Here's how the part is built. I have some questions about the finished solid (model axes, mm). A direction names the side the tool comes from. Coordinates: 2 decimals unless noted, no trailing zeros. Write each loop counter-clockwise with the first axis right and the second up, starting at its lowest first coordinate (ties: lowest second). Pieces come first, ordered by that corner, then holes.
from build123d import *

# Parameters (mm, degrees)
F0_W      = 1.2
F0_H      = 9
F5_DEPTH  = 9
F7_DEPTH  = 1
F6_W      = 6
F6_H      = 1
F8_DEPTH  = 0.4
F9_DEPTH  = 1
F6_W_2    = 1
F6_H_2    = 1.2
F10_DEPTH = 1
F11_R     = 0.3
F13_DEPTH = 1
F14_DEPTH = 0.4
F15_SIZE  = 0.2


with BuildPart() as f2:
    # F2: sweep along a path in F1
    with BuildLine(Plane.XZ) as f2_path:
        Line((0, 0), (0, 1))
    # F0 (on Top) → F2 (sweep)
    with BuildSketch(Plane.XY):
        Polygon((-12, -8), (12, -8), (12, 1), (12, 8), (12, 9), (12, 17), (-12, 17), (-12, 9), (-12, 8), (-12, 1), align=None)
        with Locations((-12.6, -3.5)):
            Rectangle(F0_W, F0_H)
        with Locations((12.6, -3.5)):
            Rectangle(F0_W, F0_H)
    sweep(path=f2_path.line)

    # F3: sweep along a path in F1
    with BuildLine(Plane.XZ) as f3_path:
        Line((0, 0), (0, 1))
        Line((0, 1), (0, 4))
    # F0 (on Top) → F3 (sweep)
    with BuildSketch(Plane.XY):
        with Locations((-12.6, -3.5)):
            Rectangle(F0_W, F0_H)
        with Locations((12.6, -3.5)):
            Rectangle(F0_W, F0_H)
    sweep(path=f3_path.line)

    # F4 (on face) → F5 (join, through all)
    with BuildSketch(Plane.XZ.offset(8)):
        Polygon((-11.75, 1), (-12, 4), (-12, 1), align=None)
        Polygon((12, 1), (12, 4), (11.75, 1), align=None)
    extrude(amount=-F5_DEPTH)

    # F6 (on face) → F7 (join)
    with BuildSketch(Plane.XY.offset(1)):
        Polygon((-11, 17), (-12, 17), (-12, 15.8), (-12, 9), (-11, 9), (-11, 16), align=None)
        Polygon((9, 17), (0, 17), (0, 16), (8, 16), (8, 10), (9, 10), align=None)
    extrude(amount=F7_DEPTH)

    # F6 (on face) → F8 (join)
    with BuildSketch(Plane.XY.offset(1)):
        with Locations((-8, 16.5)):
            Rectangle(F6_W, F6_H)
    extrude(amount=F8_DEPTH)

    # F6 (on face) → F9 (cut, through all)
    with BuildSketch(Plane.XY.offset(1)):
        with BuildLine():
            ThreePointArc((-7.9, 14.5), (-9.4, 13), (-7.9, 11.5))
            Line((-7.9, 11.5), (4.9, 11.5))
            ThreePointArc((4.9, 11.5), (6.4, 13), (4.9, 14.5))
            Line((4.9, 14.5), (-7.9, 14.5))
        make_face()
        with BuildLine():
            Line((12, 11.5), (12, 14.5))
            ThreePointArc((12, 14.5), (10.5, 13), (12, 11.5))
        make_face()
    extrude(amount=-F9_DEPTH, mode=Mode.SUBTRACT)

    # F6 (on face) → F10 (join, through all)
    with BuildSketch(Plane.XY.offset(1)):
        with Locations((-12.5, 16.4)):
            Rectangle(F6_W_2, F6_H_2)
    extrude(amount=-F10_DEPTH)

    # F11
    f11_edges = [f2.edges().sort_by_distance(p)[0] for p in [
        (-11.875, -8, 2.5),
        (-11.875, 1, 2.5),
        (11.875, -8, 2.5),
        (-11, 9, 1.5),
        (0, 16, 1.5),
        (0, 17, 1.5),
        (8, 10, 1.5),
        (9, 10, 1.5),
        (-12, 9, 1.5),
        (-12, 17, 1.5),
        (-13, 17, 0.5),
        (-5, 16, 1.2),
        (-5, 17, 1.2),
        (11.875, 1, 2.5),
    ]]
    fillet(f11_edges, radius=F11_R)

    # F12 (on face) → F13 (cut, through all)
    with BuildSketch(Plane.XY.offset(1)):
        with BuildLine():
            ThreePointArc((8, 15.9), (8.0707106781, 15.9292893219), (8.1, 16))
            ThreePointArc((8.1, 16), (8, 16.1), (7.9, 16))
            Line((7.9, 16), (8, 16))
            Line((8, 16), (8, 15.9))
        make_face()
    extrude(amount=F13_DEPTH, mode=Mode.SUBTRACT)

    # F12 (on face) → F14 (cut, through all)
    with BuildSketch(Plane.XY.offset(1)):
        with BuildLine():
            Line((-11, 16), (-10.9, 16))
            ThreePointArc((-10.9, 16), (-11.0707106781, 16.0707106781), (-11, 15.9))
            Line((-11, 15.9), (-11, 16))
        make_face()
    extrude(amount=F14_DEPTH, mode=Mode.SUBTRACT)

    # F15
    f15_edges = [f2.edges().sort_by_distance(p)[0] for p in [
        (-0.35, 17, 0),
        (-12.912132, 16.912132, 0),
        (12, 15.75, 0),
        (-13, 16.25, 0),
        (10.5, 13, 0),
        (-12.5, 15.8, 0),
        (12, 6.25, 0),
        (-12, 8.4, 0),
        (12.6, 1, 0),
        (-12.6, 1, 0),
        (13.2, -3.5, 0),
        (-13.2, -3.5, 0),
        (0, -8, 0),
        (-9.4, 13, 0),
        (-1.5, 14.5, 0),
        (6.4, 13, 0),
        (-1.5, 11.5, 0),
    ]]
    chamfer(f15_edges, length=F15_SIZE)


solid = f2.part
1. For pin 1 Ø3.5 at (x, y) = (3.5, 13) entering from +Z; pin 2 Ø0.5 at (y, z) = (13, 1.5) entering from -X; pin 3 Ø0.6 at (x, z) = (13, 2) entering from +Y, each with a flat end and sliding along its axis, tell me the tip position at first contact or that it passes through.
2. I want a section at A-A (x = -2). List the corners of the cut face in (y, z) for me, then the cut area to 3 significant figures.
3. Thinking about a two-plate mould opening in X: for faces 6 (the face through (12, 6.2, 0.6)), 7 (the face through (-11.873, -3.559, 2.479)), 8 (the face through (-11.5, 13.1, 2)), which applies, pulls with the +X half, pulls with the -X half, needs draft (parallel to the pull), parting line crosses it, or undercut?
4. I want a section at D-D (x = 9.75). List the corners of the cut face in (y, z) for me.
5. On a 3-axis mill with a long thin cutter (end or side, diameter ignored), from which of +Z, -Z, +X, -X, +Y, -Y can I reach the whole of each face in a straight line? I mean faces 1 (the face through (13, 1, 2)), 2 (the face through (4, 16, 1.5)), 3 (the face through (11.877, -3.559, 2.521)), 4 (the face through (-12.5, 16.4, 1)), 5 (the face through (-9.4, 13, 0.6)). Say none if no direction works.
6. I want a section at C-C (y = 4.75). List the corners of the cut face in (x, z) for me.
7. I want a section at B-B (y = 13). List the corners of the cut face in (x, z) for me, then the cut area to 3 significant figures.
8. If I drill on line 1 (X direction, y = 16.25, z = 1.6); line 2 (Z direction, x = 5.5, y = -4.75); line 3 (Y direction, x = 3.75, z = 1.05), over which ranges is the centre line in solid material (lowest first)?
Response values:
1. pin 1: stops at z = 1
1. pin 2: stops at x = -12
1. pin 3: stops at y = 1
2. outline: (-8, 0.2) - (-7.8, 0) - (11.3, 0) - (11.5, 0.2) - (11.5, 1) - (-8, 1) - close; (14.5, 0.2) - (14.7, 0) - (16.8, 0) - (17, 0.2) - (17, 1) - (14.5, 1) - close
2. area: 21.9 mm2
3. face 6: pulls with the +X half
3. face 7: undercut
3. face 8: needs draft
4. outline: (-8, 0.2) - (-7.8, 0) - (16.8, 0) - (17, 0.2) - (17, 1) - (-8, 1) - close
5. face 1: +Z, -Z, +X, +Y
5. face 2: +Z, -Y
5. face 3: +Z, +Y, -Y
5. face 4: +Z, -X, +Y
5. face 5: +Z, -Z
6. outline: (-12, 0.2) - (-11.8, 0) - (11.8, 0) - (12, 0.2) - (12, 1) - (-12, 1) - close
7. outline: (-12, 0.2) - (-11.8, 0) - (-9.6, 0) - (-9.4, 0.2) - (-9.4, 1) - (-11, 1) - (-11, 2) - (-12, 2) - close; (6.4, 0.2) - (6.6, 0) - (10.3, 0) - (10.5, 0.2) - (10.5, 1) - (9, 1) - (9, 2) - (8, 2) - (8, 1) - (6.4, 1) - close
7. area: 8.62 mm2
8. line 1: x = -12 to -11, 0 to 9
8. line 2: z = 0 to 1
8. line 3: y = 16 to 17
